Could you check a few things on this model? Use its own coordinates, in mm. Face numbers are marked on the shaded views. A direction names the side the tool comes from. Round coordinates to 2 decimals unless told otherwise and drop trailing zeros. Write each loop counter-clockwise with the first axis right and the second up, starting at its lowest first coordinate (ties: lowest second). Pieces come first, ordered by that corner, then holes. Notation, with made-up numbers: (27, 37.5) -> (41, 37.5) arc R19 cw to (41, 56.5) -> close; hole circle Ø5 at (7.25, 32). An arc over 180 degrees is marked (long way). Return JSON: item names as keys, results as strings.
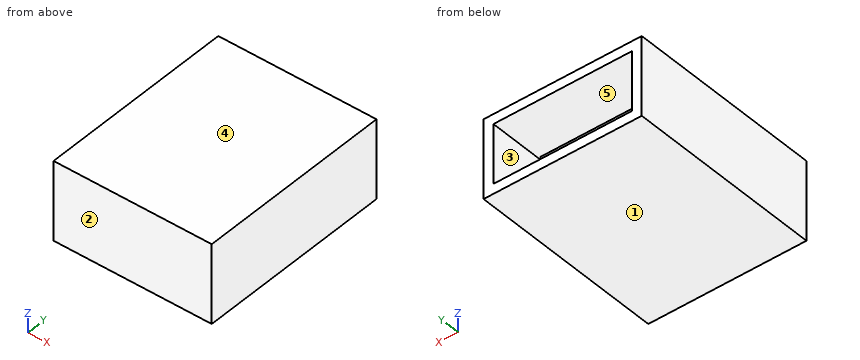
from build123d import *

# Parameters (mm, degrees)
F0_W      = 32
F0_H      = 40
F1_DEPTH  = 2
F3_W      = 22
F3_H      = 22
F4_DEPTH  = 10
F6_DEPTH  = 1
F7_DEPTH  = 1
F5_W      = 20
F5_H      = 6
F8_DEPTH  = 20
F9_W      = 12
F9_H      = 2
F10_DEPTH = 20
F11_W     = 12
F11_H     = 8
F12_DEPTH = 25
F13_W     = 14.6482707933
F13_H     = 4
F14_DEPTH = 25
F15_W     = 14
F15_H     = 14
F16_DEPTH = 5
F2_W      = 32
F2_H      = 40
F2_W_2    = 28
F2_H_2    = 36
F17_DEPTH = 14
F19_W     = 28
F19_H     = 2
F20_DEPTH = 14
F18_W     = 28
F18_H     = 2
F21_DEPTH = 38


with BuildPart() as f1:
    # F0 (on Top) → F1 (new body)
    with BuildSketch(Plane.XY):
        Rectangle(F0_W, F0_H)
    extrude(amount=F1_DEPTH)

    # F3 (on face) → F4 (join)
    with BuildSketch(Plane.XY.offset(2)):
        Rectangle(F3_W, F3_H)
    extrude(amount=F4_DEPTH)

    # F6 (add): a face of the model
    f6_faces = [f1.faces().sort_by_distance(p)[0] for p in [
        (-11, 0, 7),
    ]]
    extrude(f6_faces, amount=F6_DEPTH)

    # F7 (add): a face of the model
    f7_faces = [f1.faces().sort_by_distance(p)[0] for p in [
        (11, 0, 7),
    ]]
    extrude(f7_faces, amount=F7_DEPTH)

    # F5 (on face) → F8 (cut)
    with BuildSketch(Plane(origin=(0, 11, 0), x_dir=(-1, 0, 0), z_dir=(0, 1, 0))):
        with Locations((0, 7)):
            Rectangle(F5_W, F5_H)
    extrude(amount=-F8_DEPTH, mode=Mode.SUBTRACT)

    # F9 (on face) → F10 (cut)
    with BuildSketch(Plane(origin=(0, 11, 0), x_dir=(-1, 0, 0), z_dir=(0, 1, 0))):
        with Locations((0, 3)):
            Rectangle(F9_W, F9_H)
    extrude(amount=-F10_DEPTH, mode=Mode.SUBTRACT)

    # F11 (on face) → F12 (cut)
    with BuildSketch(Plane(origin=(-12, 0, 0), x_dir=(0, -1, 0), z_dir=(-1, 0, 0))):
        with Locations((0, 6)):
            Rectangle(F11_W, F11_H)
    extrude(amount=-F12_DEPTH, mode=Mode.SUBTRACT)

    # F13 (on face) → F14 (cut)
    with BuildSketch(Plane.XZ.offset(11)):
        with Locations((0, 6.5)):
            Rectangle(F13_W, F13_H)
    extrude(amount=-F14_DEPTH, mode=Mode.SUBTRACT)

    # F15 (on face) → F16 (cut)
    with BuildSketch(Plane.XY.offset(12)):
        Rectangle(F15_W, F15_H)
    extrude(amount=-F16_DEPTH, mode=Mode.SUBTRACT)

    # F2 (on face) → F17 (join)
    with BuildSketch(Plane.XY.offset(2)):
        Rectangle(F2_W, F2_H)
        Rectangle(F2_W_2, F2_H_2, mode=Mode.SUBTRACT)
    extrude(amount=F17_DEPTH)

    # F19 (on face) → F20 (cut)
    with BuildSketch(Plane.XY.offset(16)):
        with Locations((0, 19)):
            Rectangle(F19_W, F19_H)
    extrude(amount=-F20_DEPTH, mode=Mode.SUBTRACT)

    # F18 (on face) → F21 (join)
    with BuildSketch(Plane(origin=(0, -18, 0), x_dir=(-1, 0, 0), z_dir=(0, 1, 0))):
        with Locations((0, 15)):
            Rectangle(F18_W, F18_H)
    extrude(amount=F21_DEPTH)


solid = f1.part
1) I want a section at D-D, the plane y = -10. Please give me the cut outline in (x, z).
Return value:
{"outline": "(-16, 0) -> (16, 0) -> (16, 16) -> (-16, 16) -> close; hole (-14, 2) -> (-12, 2) -> (-12, 12) -> (12, 12) -> (12, 2) -> (14, 2) -> (14, 14) -> (-14, 14) -> close; hole (-7.32, 4.5) -> (7.32, 4.5) -> (7.32, 8.5) -> (-7.32, 8.5) -> close"}
2) Thinking about a two-plate mould opening in Z: for the marked faces 1, 2 and 3, which applies, pulls with the +Z half, pulls with the -Z half, needs draft (parallel to the pull), parting line crosses it, or undercut?
Return value:
{"face 1": "pulls with the -Z half", "face 2": "needs draft", "face 3": "undercut"}
3) I want a section at B-B, the plane y = -4.5. Please give me the cut outline in (x, z), and give its area (3 significant figures).
Return value:
{"outline": "(-16, 0) -> (16, 0) -> (16, 16) -> (-16, 16) -> close; (-12, 10) -> (-7, 10) -> (-7, 12) -> (-12, 12) -> close; (7, 10) -> (12, 10) -> (12, 12) -> (7, 12) -> close; hole (-14, 2) -> (14, 2) -> (14, 14) -> (-14, 14) -> close", "area": "196 mm²"}
4) I want a section at A-A, the plane z = 10.75. Please give me the cut outline in (x, y).
Return value:
{"outline": "(-16, -20) -> (16, -20) -> (16, 20) -> (14, 20) -> (14, -18) -> (-14, -18) -> (-14, 20) -> (-16, 20) -> close; (-12, -11) -> (12, -11) -> (12, 11) -> (-12, 11) -> close; hole (-7, -7) -> (7, -7) -> (7, 7) -> (-7, 7) -> close"}
5) For the marked faces 4 and 5, which set-ups out of +Z, -Z, +X, -X, +Y, -Y let a thin tool reach every point of the face, with its end or its side?
Return value:
{"face 4": "+Z, +X, -X, +Y, -Y", "face 5": "+Y"}
6) Will these pins go through, and if not, where does the flat tip stop? pin 1 Ø0.6 at (x, z) = (0, 11) entering from +Y; pin 2 Ø5 at (x, z) = (-1, 5.5) entering from +Y.
Return value:
{"pin 1": "y = 11", "pin 2": "y = -9"}
7) I want a section at C-C, the plane z = 2.75. Please give me the cut outline in (x, y), and give its area (3 significant figures).
Return value:
{"outline": "(-16, -20) -> (16, -20) -> (16, 20) -> (14, 20) -> (14, -18) -> (-14, -18) -> (-14, 20) -> (-16, 20) -> close; (-12, -11) -> (12, -11) -> (12, -6) -> (6, -6) -> (6, -9) -> (-6, -9) -> (-6, -6) -> (-12, -6) -> close; (-12, 6) -> (-6, 6) -> (-6, 11) -> (-12, 11) -> close; (6, 6) -> (12, 6) -> (12, 11) -> (6, 11) -> close", "area": "360 mm²"}
8) If I drill on probe 1 along Z at (x, y) = (-8, -8); probe 2 along Y at (x, z) = (9, 9.25); probe 3 along Z at (x, y) = (5, 12.5), over which ranges is the centre line in solid material (lowest first)? Write a range as [from, to].
Return value:
{"probe 1": "[0, 4], [10, 12], [14, 16]", "probe 2": "[-20, -18], [-11, -9]", "probe 3": "[0, 2], [14, 16]"}
